The model under review builds one solid part; all positions refer to its coordinate system, in mm. A direction names the side the tool comes from. Coordinates: 2 decimals unless noted, no trailing zeros. Loops run counter-clockwise (first coordinate to the right, second up) from the corner with the lowest first, then second, coordinate; pieces in that order, holes last. Notation, with made-up numbers: (29.25, 2) - (57.25, 2) arc R18 cw to (57.25, 14) - close; hole circle Ø1 at (83, 26). An arc over 180 degrees is marked (long way). Use a Markdown table: item, result. Add a question column.
1) The part is to be moulded in two halves that separate along Y. For faces 1 (the cylindrical face through (-7.416, 9.681, 12.522)), 2 (the cylindrical face through (-3.53, -12.14, 12.52)), 3 (the flat face through (5.67, -7.05, 12.52)), 4 (the flat face through (3, 0, 25.4)), say which applies: pulls with the +Y half, pulls with the -Y half, needs draft (parallel to the pull), parting line crosses it, or undercut.
2) Add section D-D, the plane x = 9.25. Give the boundary of the cut face in (y, z).
3) For faces 5 (the flat face through (7.07, 5.763, 12.522)), 6 (the cylindrical face through (3.52, -12.13, 12.52)), 7 (the cylindrical face through (3.53, 12.14, 12.52)), list the 3-axis set-ups (+Z, -Z, +X, -X, +Y, -Y) from which the entire face can be reached by the end or side of a thin tool; tool diameter is ignored.
4) Add section A-A, the plane y = -1. Give the boundary of the cut face in (x, z), and give its area (3 significant figures).
5) Add section C-C, the plane y = 9. Give the boundary of the cut face in (x, z), and give its area (3 significant figures).
6) Clearance check with flat-ended pins moving along their axes: pin 1 (1.5 mm diameter, centred on x = 5.5, z = 11.5, fed in from -Y); pin 2 (3 mm diameter, centred on x = -0.5, z = 7.5, fed in from +Y); pin 3 (10 mm diameter, centred on x = 7.5, z = 13, fed in from -Y); pin 4 (0.8 mm diameter, centred on x = 0, z = 7, fed in from -Y). State where each tip first meets the part, or that it passes through.
7) Add section B-B, the plane x = 6. Give the boundary of the cut face in (y, z).
8) To check wall thickness, follow L1, parallel to X at y = -2, z = 3; L2, parallel to X at y = -4, z = 14.25; L3, parallel to Y at x = 5.5, z = 11. State the ranges of each line that lie inside material, in increasing order. Write a range as [from, to].
```python
from build123d import *

# Parameters (mm, degrees)
EXTRUDE1_DEPTH = 25.4


with BuildPart() as part:
    # Sketch1 → Extrude1 (new body)
    with BuildSketch(Plane.XY):
        with BuildLine():
            Line((11.125675541, 12.699168884), (4.22095036, 12.445641481))
            ThreePointArc((4.22095036, 12.445641481), (3.524314259, 12.136654887), (3.2385, 11.430195559))
            Line((3.2385, 11.430195559), (3.2385, 11.226884683))
            ThreePointArc((3.2385, 11.226884683), (3.548040671, 10.496698941), (4.28804964, 10.21143876))
            Line((4.28804964, 10.21143876), (6.44345036, 10.308051727))
            ThreePointArc((6.44345036, 10.308051727), (7.4091133, 9.696859185), (7.19542049, 8.574185315))
            Line((7.19542049, 8.574185315), (4.193053216, 5.571818041))
            ThreePointArc((4.193053216, 5.571818041), (2.874596726, 4.69085358), (1.319371257, 4.3815))
            Line((1.319371257, 4.3815), (-1.319371257, 4.3815))
            ThreePointArc((-1.319371257, 4.3815), (-2.874596726, 4.69085358), (-4.193053216, 5.571818041))
            Line((-4.193053216, 5.571818041), (-7.19542049, 8.574185315))
            ThreePointArc((-7.19542049, 8.574185315), (-7.4091133, 9.696859185), (-6.44345036, 10.308051727))
            Line((-6.44345036, 10.308051727), (-4.28804964, 10.21143876))
            ThreePointArc((-4.28804964, 10.21143876), (-3.548040671, 10.496698941), (-3.2385, 11.226884683))
            Line((-3.2385, 11.226884683), (-3.2385, 11.430195559))
            ThreePointArc((-3.2385, 11.430195559), (-3.524314259, 12.136654887), (-4.22095036, 12.445641481))
            Line((-4.22095036, 12.445641481), (-11.125675541, 12.699168884))
            ThreePointArc((-11.125675541, 12.699168884), (-12.235688993, 12.271278612), (-12.7, 11.176))
            Line((-12.7, 11.176), (-12.7, 0))
            Line((-12.7, 0), (-12.7, -11.176))
            ThreePointArc((-12.7, -11.176), (-12.235688993, -12.271278612), (-11.125675541, -12.699168884))
            Line((-11.125675541, -12.699168884), (-4.22095036, -12.445641481))
            ThreePointArc((-4.22095036, -12.445641481), (-3.524314259, -12.136654887), (-3.2385, -11.430195559))
            Line((-3.2385, -11.430195559), (-3.2385, -11.226884683))
            ThreePointArc((-3.2385, -11.226884683), (-3.548040671, -10.496698941), (-4.28804964, -10.21143876))
            Line((-4.28804964, -10.21143876), (-6.44345036, -10.308051727))
            ThreePointArc((-6.44345036, -10.308051727), (-7.4091133, -9.696859185), (-7.19542049, -8.574185315))
            Line((-7.19542049, -8.574185315), (-4.193053216, -5.571818041))
            ThreePointArc((-4.193053216, -5.571818041), (-2.874596726, -4.69085358), (-1.319371257, -4.3815))
            Line((-1.319371257, -4.3815), (1.319371257, -4.3815))
            ThreePointArc((1.319371257, -4.3815), (2.874596726, -4.69085358), (4.193053216, -5.571818041))
            Line((4.193053216, -5.571818041), (7.19542049, -8.574185315))
            ThreePointArc((7.19542049, -8.574185315), (7.4091133, -9.696859185), (6.44345036, -10.308051727))
            Line((6.44345036, -10.308051727), (4.28804964, -10.21143876))
            ThreePointArc((4.28804964, -10.21143876), (3.548040671, -10.496698941), (3.2385, -11.226884683))
            Line((3.2385, -11.226884683), (3.2385, -11.430195559))
            ThreePointArc((3.2385, -11.430195559), (3.524314259, -12.136654887), (4.22095036, -12.445641481))
            Line((4.22095036, -12.445641481), (11.125675541, -12.699168884))
            ThreePointArc((11.125675541, -12.699168884), (12.235688993, -12.271278612), (12.7, -11.176))
            Line((12.7, -11.176), (12.7, 0))
            Line((12.7, 0), (12.7, 11.176))
            ThreePointArc((12.7, 11.176), (12.235688993, 12.271278612), (11.125675541, 12.699168884))
        make_face()
        with BuildLine():
            Line((-8.50177951, 7.19542049), (-5.597218041, 4.290859021))
            ThreePointArc((-5.597218041, 4.290859021), (-4.71625358, 2.972402531), (-4.4069, 1.417177062))
            Line((-4.4069, 1.417177062), (-4.4069, -1.417177062))
            ThreePointArc((-4.4069, -1.417177062), (-4.71625358, -2.972402531), (-5.597218041, -4.290859021))
            Line((-5.597218041, -4.290859021), (-8.50177951, -7.19542049))
            ThreePointArc((-8.50177951, -7.19542049), (-9.609006367, -7.415661605), (-10.2362, -6.477))
            Line((-10.2362, -6.477), (-10.2362, 0))
            Line((-10.2362, 0), (-10.2362, 6.477))
            ThreePointArc((-10.2362, 6.477), (-9.609006367, 7.415661605), (-8.50177951, 7.19542049))
        make_face(mode=Mode.SUBTRACT)
        with BuildLine():
            Line((10.2362, 0), (10.2362, 6.477))
            ThreePointArc((10.2362, 6.477), (9.609006367, 7.415661605), (8.50177951, 7.19542049))
            Line((8.50177951, 7.19542049), (5.597218041, 4.290859021))
            ThreePointArc((5.597218041, 4.290859021), (4.71625358, 2.972402531), (4.4069, 1.417177062))
            Line((4.4069, 1.417177062), (4.4069, -1.417177062))
            ThreePointArc((4.4069, -1.417177062), (4.71625358, -2.972402531), (5.597218041, -4.290859021))
            Line((5.597218041, -4.290859021), (8.50177951, -7.19542049))
            ThreePointArc((8.50177951, -7.19542049), (9.609006367, -7.415661605), (10.2362, -6.477))
            Line((10.2362, -6.477), (10.2362, 0))
        make_face(mode=Mode.SUBTRACT)
        with BuildLine():
            ThreePointArc((0, 2.5527), (-1.80503148, 1.80503148), (-2.5527, 0))
            ThreePointArc((-2.5527, 0), (-1.80503148, -1.80503148), (0, -2.5527))
            ThreePointArc((0, -2.5527), (1.80503148, -1.80503148), (2.5527, 0))
            ThreePointArc((2.5527, 0), (1.80503148, 1.80503148), (0, 2.5527))
        make_face(mode=Mode.SUBTRACT)
    extrude(amount=EXTRUDE1_DEPTH)


solid = part.part
```
From the geometry:
| question | item | result |
|---|---|---|
| 1 | face 1 | undercut |
| 1 | face 2 | pulls with the -Y half |
| 1 | face 3 | undercut |
| 1 | face 4 | needs draft |
| 2 | outline | (-12.63, 0) - (-7.49, 0) - (-7.49, 25.4) - (-12.63, 25.4) - close; (7.49, 0) - (12.63, 0) - (12.63, 25.4) - (7.49, 25.4) - close |
| 3 | face 5 | +Z, -Z |
| 3 | face 6 | +Z, -Z, -Y |
| 3 | face 7 | +Z, -Z, +Y |
| 4 | outline | (-12.7, 0) - (-10.24, 0) - (-10.24, 25.4) - (-12.7, 25.4) - close; (-4.41, 0) - (-2.35, 0) - (-2.35, 25.4) - (-4.41, 25.4) - close; (2.35, 0) - (4.41, 0) - (4.41, 25.4) - (2.35, 25.4) - close; (10.24, 0) - (12.7, 0) - (12.7, 25.4) - (10.24, 25.4) - close |
| 4 | area | 230 mm^2 |
| 5 | outline | (-12.7, 0) - (-7.45, 0) - (-7.45, 25.4) - (-12.7, 25.4) - close; (7.45, 0) - (12.7, 0) - (12.7, 25.4) - (7.45, 25.4) - close |
| 5 | area | 267 mm^2 |
| 6 | pin 1 | stops at y = -12.52 |
| 6 | pin 2 | stops at y = 4.44 |
| 6 | pin 3 | stops at y = -12.7 |
| 6 | pin 4 | stops at y = -4.38 |
| 7 | outline | (-12.51, 0) - (-10.29, 0) - (-10.29, 25.4) - (-12.51, 25.4) - close; (-7.38, 0) - (-4.69, 0) - (-4.69, 25.4) - (-7.38, 25.4) - close; (4.69, 0) - (7.38, 0) - (7.38, 25.4) - (4.69, 25.4) - close; (10.29, 0) - (12.51, 0) - (12.51, 25.4) - (10.29, 25.4) - close |
| 8 | L1 | x = [-12.7, -10.24], [-4.45, -1.59], [1.59, 4.45], [10.24, 12.7] |
| 8 | L2 | x = [-12.7, -10.24], [-5.33, 5.33], [10.24, 12.7] |
| 8 | L3 | y = [-12.49, -10.27], [-6.88, -4.19], [4.19, 6.88], [10.27, 12.49] |
